Build history of the part. All positions in model axes, mm. A direction names the side the tool comes from. Give positions to 0.01 mm unless a question says otherwise; leave off trailing zeros. Write each loop counter-clockwise with the first axis right and the second up, starting at its lowest first coordinate (ties: lowest second). Pieces come first, ordered by that corner, then holes. Notation, with made-up numbers: (51, -37) -> (92, -37) arc R15 cw to (92, -31) -> close; hole circle Ø3 at (66.25, -39). An arc over 180 degrees is marked (long way). One line per question, with ' | ' between items. Start each with the question number.
(1) Band-saw the part on B-B, the plane y = 0. Give the cut face in (x, z).
(2) Pin check, flat tips, straight feed: P1, Ø13.5, axis at x = 0, y = 0, coming from the +Z side; P2, Ø6, axis at x = 12.5, z = 6.5, coming from the -Y side; P3, Ø1, axis at y = -5, z = 17.5, coming from the -X side; P4, Ø19.5, axis at x = 0, y = 0, coming from the -Z side. Stop position of each tip, or through.
(3) Band-saw the part on D-D, the plane x = 6.5. Give the cut face in (y, z).
(4) Drill centre lines: probe 1 along X at (y, z) = (-0.5, -29); probe 2 along Y at (x, z) = (0, 46); probe 3 along Z at (x, y) = (22, -9). Where is each one in solid material? Low to high. Write a range as from..to.
(5) Pull direction Z, two halves, no side cores. Call faces 1 (the flat face through (40, 13.4, 20.2)), 2 (the cylindrical face through (17, 0, 20)), 3 (the flat face through (8, 4, 66)): released by +Z, released by -Z, zero draft, split by the parting line, or undercut.
(6) Band-saw the part on C-C, the plane z = 22. Give the cut face in (x, y), and give its area (3 significant figures).
(7) Band-saw the part on A-A, the plane x = 0. Give the cut face in (y, z).
(8) Tool access for faces 4 (the flat face through (8, -4, -45)), 5 (the cylindrical face through (27.332, -5.745, 6.292)): list every direction of +Z, -Z, +X, -X, +Y, -Y with a clear straight run to the whole face (end or side of a thin tool).
from build123d import *

# Parameters (mm, degrees)
SKETCH1_R           = 17
BOSS_EXTRUDE2_DEPTH = 40
SKETCH2_R           = 8.5
CUT_EXTRUDE1_DEPTH  = 38
CUT_EXTRUDE2_START  = -38
SKETCH3_R           = 8.5
CUT_EXTRUDE2_DEPTH  = 38
SKETCH4_R           = 15
SKETCH4_R_2         = 13
BOSS_EXTRUDE3_DEPTH = 40
CUT_EXTRUDE4_START  = -50
SKETCH6_R           = 8.5
CUT_EXTRUDE4_DEPTH  = 50
BOSS_EXTRUDE4_START = 45
SKETCH7_R           = 17
SKETCH7_R_2         = 8.5
BOSS_EXTRUDE4_DEPTH = 45
SKETCH8_R           = 17
SKETCH8_R_2         = 8.5
BOSS_EXTRUDE5_DEPTH = 26


with BuildPart() as part:
    # Sketch1 → Boss-Extrude2 (new body)
    with BuildSketch(Plane.XY):
        Circle(SKETCH1_R)
    extrude(amount=BOSS_EXTRUDE2_DEPTH)

    # Sketch2 → Cut-Extrude1 (cut)
    with BuildSketch(Plane.XY.offset(40)):
        Circle(SKETCH2_R)
    extrude(amount=-CUT_EXTRUDE1_DEPTH, mode=Mode.SUBTRACT)

    # Sketch3 → Cut-Extrude2 (cut)
    with BuildSketch(Plane(origin=(0, 0, 0), x_dir=(-1, 0, 0), z_dir=(0, 0, -1)).offset(CUT_EXTRUDE2_START)):
        with Locations(Location((0, 0, 0), (0, 0, 180))):
            Circle(SKETCH3_R)
    extrude(amount=CUT_EXTRUDE2_DEPTH, mode=Mode.SUBTRACT)

    # Sketch4 → Boss-Extrude3 (add)
    with BuildSketch(Plane(origin=(0, 0, 0), x_dir=(0, 0, -1), z_dir=(1, 0, 0))):
        with Locations((-20.148533522, 0)):
            Circle(SKETCH4_R)
        with Locations(Location((-20.148533522, 0, 0), (0, 0, 180))):
            Circle(SKETCH4_R_2, mode=Mode.SUBTRACT)
    extrude(amount=BOSS_EXTRUDE3_DEPTH)

    # Sketch6 → Cut-Extrude4 (cut)
    with BuildSketch(Plane(origin=(0, 0, 0), x_dir=(-1, 0, 0), z_dir=(0, 0, -1)).offset(CUT_EXTRUDE4_START)):
        with Locations(Location((0, 0, 0), (0, 0, 180))):
            Circle(SKETCH6_R)
    extrude(amount=CUT_EXTRUDE4_DEPTH, mode=Mode.SUBTRACT)

    # Sketch7 → Boss-Extrude4 (add)
    with BuildSketch(Plane(origin=(0, 0, 0), x_dir=(-1, 0, 0), z_dir=(0, 0, -1)).offset(BOSS_EXTRUDE4_START)):
        Circle(SKETCH7_R)
        with Locations(Location((0, 0, 0), (0, 0, 180))):
            Circle(SKETCH7_R_2, mode=Mode.SUBTRACT)
    extrude(amount=-BOSS_EXTRUDE4_DEPTH)

    # Sketch8 → Boss-Extrude5 (add)
    with BuildSketch(Plane.XY.offset(40)):
        with Locations(Location((0, 0, 0), (0, 0, 180))):
            Circle(SKETCH8_R)
        Circle(SKETCH8_R_2, mode=Mode.SUBTRACT)
    extrude(amount=BOSS_EXTRUDE5_DEPTH)


solid = part.part
Results:
1) outline: (-17, -45) -> (-8.5, -45) -> (-8.5, 66) -> (-17, 66) -> close; (8.5, -45) -> (17, -45) -> (17, 5.15) -> (40, 5.15) -> (40, 7.15) -> (17, 7.15) -> (17, 33.15) -> (40, 33.15) -> (40, 35.15) -> (17, 35.15) -> (17, 66) -> (8.5, 66) -> close
2) P1: passes through | P2: stops at y = -14.1 | P3: stops at x = -16.39 | P4: stops at z = -45
3) outline: (-15.71, -45) -> (-5.48, -45) -> (-5.48, 66) -> (-15.71, 66) -> close; (5.48, -45) -> (15.71, -45) -> (15.71, 66) -> (5.48, 66) -> close
4) probe 1: x = -16.99..-8.49, 8.49..16.99 | probe 2: y = -17..-8.5, 8.5..17 | probe 3: z = 8.15..10.77, 29.53..32.15
5) face 1: zero draft | face 2: undercut | face 3: released by +Z
6) outline: (8.21, -14.89) -> (40, -14.89) -> (40, -12.87) -> (11.11, -12.87) arc R17 ccw to (11.11, 12.87) -> (40, 12.87) -> (40, 14.89) -> (8.21, 14.89) arc R17 ccw (long way) to start; hole circle Ø17 at (0, 0) | area: 803 mm²
7) outline: (-17, -45) -> (-8.5, -45) -> (-8.5, 66) -> (-17, 66) -> close; (8.5, -45) -> (17, -45) -> (17, 66) -> (8.5, 66) -> close
8) face 4: -Z, +X, -X, +Y, -Y | face 5: +X
